Model file for the job. Use its own axes, mm. A direction names the side the tool comes from. Give positions to 0.01 mm unless a question says otherwise; leave off trailing zeros. Loops run counter-clockwise (first coordinate to the right, second up) from the corner with the lowest first, then second, coordinate; pieces in that order, holes last. Notation, with made-up numbers: (60.5, 29.25) - (74.5, 29.25) arc R23 cw to (74.5, 68.25) - close; hole circle Ø2 at (-19, -36). An arc over 180 degrees is marked (long way). Answer as CSV lines item,"result". Start each with the question number.
Item 1: Saw through at B-B on z = 27. Give the cut face in (x, y), plus the area to 3 significant figures.
Item 2: Tool access for faces 1 (the flat face through (-159, -5, 48)), 2 (the flat face through (-159, 0.5, 36)), 3 (the cylindrical face through (-164.929, -3.958, 7.93)): list every direction of +Z, -Z, +X, -X, +Y, -Y with a clear straight run to the whole face (end or side of a thin tool).
Item 3: Drill centre lines: L1, parallel to Z at x = -150.75, y = -2.5; L2, parallel to Y at x = -154.75, z = 36.5; L3, parallel to Y at x = -161.75, z = 34.5. Where is each one in solid material? Low to high. Write a range as from..to.
Item 4: Saw through at C-C on y = -1. Give the cut face in (x, z), plus the area to 3 significant figures.
Item 5: Pull direction Y, two halves, no side cores. Call faces 4 (the cylindrical face through (-153.071, -1.042, 7.93)), 5 (the flat face through (-159, 3.5, 25)), 6 (the cylindrical face through (-164.929, -1.042, 25.367)), 7 (the flat face through (-159, -5, 3)): pulls with the +Y half, pulls with the -Y half, needs draft (parallel to the pull), parting line crosses it, or undercut.
Item 6: Saw through at D-D on x = -153.25. Give the cut face in (y, z), plus the area to 3 significant figures.
Item 7: Saw through at A-A on x = -159. Give the cut face in (y, z), plus the area to 3 significant figures.
from build123d import *

# Parameters (mm, degrees)
BOX166_W               = 6
BOX166_H               = 26
BOX166_DEPTH           = 3
BOX165_W               = 4
BOX165_H               = 53
BOX165_DEPTH           = 13
FILLET020_R            = 1.9
BOX164_W               = 6
BOX164_H               = 26
BOX164_DEPTH           = 3
BOX163_W               = 12
BOX163_H               = 21
BOX163_DEPTH           = 45
CHAMFER064_1_SIZE2     = 2
CHAMFER064_1_SIZE      = 4
CHAMFER064_2_SIZE2     = 2
CHAMFER064_2_SIZE      = 4
CUT060_PLACEMENT_ANGLE = 90


with BuildPart() as cube166:
    # Box166 → Box166 (new body)
    with BuildSketch(Plane(origin=(2, -2.5, 35), x_dir=(1, 0, 0), z_dir=(0, 0, 1))):
        with Locations((3, 13)):
            Rectangle(BOX166_W, BOX166_H)
    extrude(amount=BOX166_DEPTH)


with BuildPart() as fillet020:
    # Box165 → Box165 (new body)
    with BuildSketch(Plane(origin=(3, 4, 50), x_dir=(1, 0, 0), z_dir=(0, 1, 0))):
        with Locations((2, 26.5)):
            Rectangle(BOX165_W, BOX165_H)
    extrude(amount=BOX165_DEPTH)

    # Fillet020
    fillet020_edges = [fillet020.edges().sort_by_distance(p)[0] for p in [
        (3, 17, 23.5),
        (3, 4, 23.5),
        (7, 17, 23.5),
        (7, 4, 23.5),
    ]]
    fillet(fillet020_edges, radius=FILLET020_R)


with BuildPart() as fusion086:
    # Box164 → Box164 (new body)
    with BuildSketch(Plane(origin=(2, -2.5, 13), x_dir=(1, 0, 0), z_dir=(0, 0, 1))):
        with Locations((3, 13)):
            Rectangle(BOX164_W, BOX164_H)
    extrude(amount=BOX164_DEPTH)

    # Fusion086: union Cube166, Fillet020
    add(cube166.part)
    add(fillet020.part)


with BuildPart() as obj1:
    # Box163 → Box163 (new body)
    with BuildSketch(Plane(origin=(-1, 0, 3), x_dir=(1, 0, 0), z_dir=(0, 0, 1))):
        with Locations((6, 10.5)):
            Rectangle(BOX163_W, BOX163_H)
    extrude(amount=BOX163_DEPTH)

    # Chamfer064 1
    chamfer064_1_edges = [obj1.edges().sort_by_distance(p)[0] for p in [
        (11, 0, 25.5),
        (11, 21, 25.5),
    ]]
    chamfer064_1_side = obj1.faces().sort_by_distance((11, 10.5, 25.5))[0]
    chamfer(chamfer064_1_edges, length=CHAMFER064_1_SIZE, length2=CHAMFER064_1_SIZE2, reference=chamfer064_1_side)

    # Chamfer064 2
    chamfer064_2_edges = [obj1.edges().sort_by_distance(p)[0] for p in [
        (-1, 0, 25.5),
        (-1, 21, 25.5),
    ]]
    chamfer064_2_side = obj1.faces().sort_by_distance((-1, 10.5, 25.5))[0]
    chamfer(chamfer064_2_edges, length=CHAMFER064_2_SIZE, length2=CHAMFER064_2_SIZE2, reference=chamfer064_2_side)

    # Cut060: cut Fusion086
    add(fusion086.part, mode=Mode.SUBTRACT)


with BuildPart() as obj1_1:
    # Cut060 placement: moved
    add(obj1.part.moved(Location((-169.5, 2.5, 0))).rotate(Axis((-169.5, 2.5, 0), (0, 0, -1)), CUT060_PLACEMENT_ANGLE))


solid = obj1_1.part
Responses:
1,outline,"(-169.5, -6.5) - (-165.5, -8.5) - (-152.5, -8.5) - (-148.5, -6.5) - (-148.5, 1.5) - (-152.5, 3.5) - (-165.5, 3.5) - (-169.5, 1.5) - close; hole (-165.5, -2.6) arc R1.9 ccw to (-163.6, -4.5) - (-154.4, -4.5) arc R1.9 ccw to (-152.5, -2.6) - (-152.5, -2.4) arc R1.9 ccw to (-154.4, -0.5) - (-163.6, -0.5) arc R1.9 ccw to (-165.5, -2.4) - close"
1,area,"187 mm2"
2,face 1,"+Z, +X, -X, +Y, -Y"
2,face 2,"+X, -X"
2,face 3,"+Z, -Z"
3,L1,"3..13, 16..35, 38..48"
3,L2,"-8.5..-5.5, 0.5..3.5"
3,L3,"-8.5..-4.5, -0.5..3.5"
4,outline,"(-169.5, 3) - (-164.88, 3) - (-164.88, 13) - (-169.5, 13) - close; (-169.5, 16) - (-164.88, 16) - (-164.88, 35) - (-169.5, 35) - close; (-169.5, 38) - (-164.88, 38) - (-164.88, 48) - (-169.5, 48) - close; (-153.12, 3) - (-148.5, 3) - (-148.5, 13) - (-153.12, 13) - close; (-153.12, 16) - (-148.5, 16) - (-148.5, 35) - (-153.12, 35) - close; (-153.12, 38) - (-148.5, 38) - (-148.5, 48) - (-153.12, 48) - close"
4,area,"360 mm2"
5,face 4,"undercut"
5,face 5,"pulls with the +Y half"
5,face 6,"undercut"
5,face 7,"needs draft"
6,outline,"(-8.5, 3) - (-4.11, 3) - (-4.11, 13) - (-5.5, 13) - (-5.5, 16) - (-4.11, 16) - (-4.11, 35) - (-5.5, 35) - (-5.5, 38) - (-4.11, 38) - (-4.11, 48) - (-8.5, 48) - close; (-0.89, 3) - (3.5, 3) - (3.5, 48) - (-0.89, 48) - (-0.89, 38) - (0.5, 38) - (0.5, 35) - (-0.89, 35) - (-0.89, 16) - (0.5, 16) - (0.5, 13) - (-0.89, 13) - close"
6,area,"378 mm2"
7,outline,"(-8.5, 3) - (-4.5, 3) - (-4.5, 13) - (-5.5, 13) - (-5.5, 16) - (-4.5, 16) - (-4.5, 35) - (-5.5, 35) - (-5.5, 38) - (-4.5, 38) - (-4.5, 48) - (-8.5, 48) - close; (-0.5, 3) - (3.5, 3) - (3.5, 48) - (-0.5, 48) - (-0.5, 38) - (0.5, 38) - (0.5, 35) - (-0.5, 35) - (-0.5, 16) - (0.5, 16) - (0.5, 13) - (-0.5, 13) - close"
7,area,"348 mm2"
